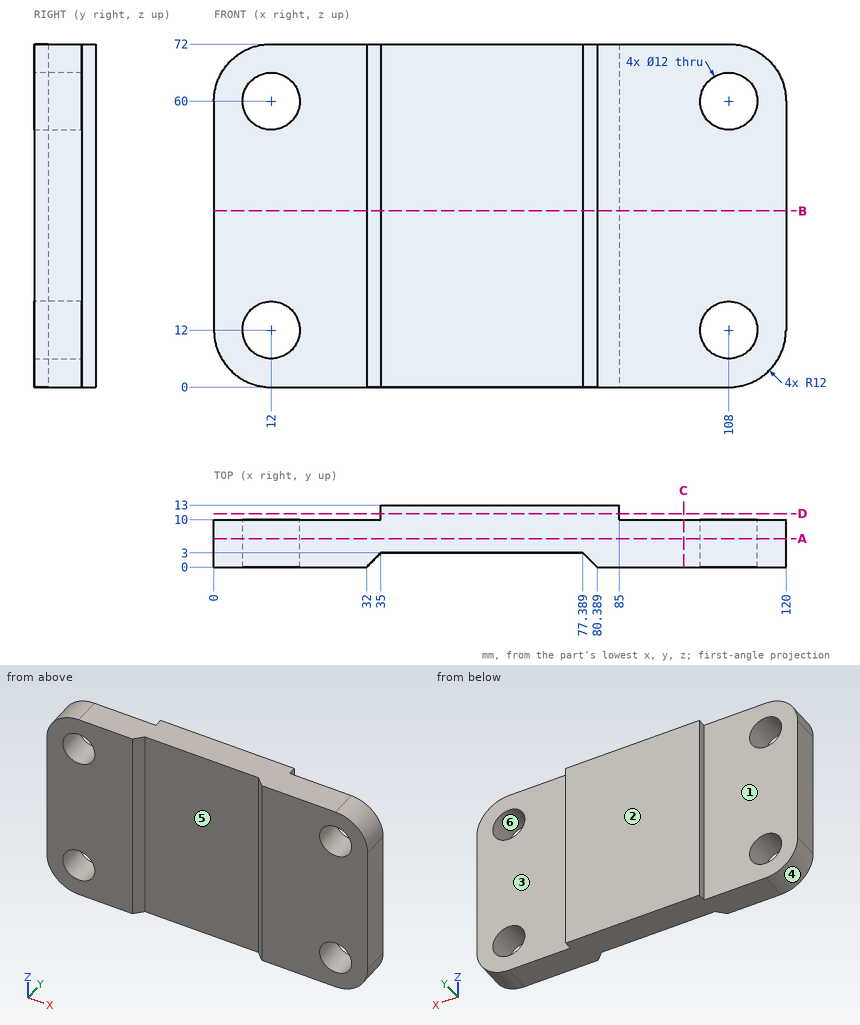
Study the drawing (mm; zero at the part's minimum x, y, z) and answer. A direction names the side the tool comes from. Give positions to 0.01 mm unless a question says otherwise; leave off trailing zeros. Order: outer loops, then holes, each group sorted by start corner. A loop starts at its lowest first (then second) coordinate and runs counter-clockwise, first axis right, second up. Notation, with made-up numbers: (86, -14.75) -> (133, -14.75) arc R23 ccw to (133, 17.25) -> close; hole circle Ø2 at (41, -32.75). An arc over 180 degrees is marked (long way). Write item = value, one per line.
1. A cutting plane is placed at C-C, the plane x = 98.5. Write down the section's boundary in (y, z), and give its area (3 significant figures).
Numbers:
outline = (0, 0) -> (10, 0) -> (10, 72) -> (0, 72) -> close
area = 720 mm²
2. The mould has two halves that part along Z. Classify the marked faces 4, 5 and 6: +Z half, -Z half, draft (parallel to the pull), parting line (faces both ways), or undercut.
Numbers:
face_4 = -Z half
face_5 = draft
face_6 = undercut
3. A cutting plane is placed at D-D, the plane y = 11.25. Write down the section's boundary in (x, z).
Numbers:
outline = (35, 0) -> (85, 0) -> (85, 72) -> (35, 72) -> close
4. A cutting plane is placed at B-B, the plane z = 37. Write down the section's boundary in (x, y), and give its area (3 significant figures).
Numbers:
outline = (0, 0) -> (32, 0) -> (35, 3) -> (77.39, 3) -> (80.39, 0) -> (120, 0) -> (120, 10) -> (85, 10) -> (85, 13) -> (35, 13) -> (35, 10) -> (0, 10) -> close
area = 1,210 mm²
5. Straight lines are drawn through the part: line 1 along Z through (x, y) = (108.5, 3.5); line 2 along Z through (x, y) = (11, 6.5); line 3 along Y through (x, z) = (38, 37.5). For each, find the intervals that lie inside material, in ascending order.
Numbers:
line_1 = 0.01 to 6.02, 17.98 to 54.02, 65.98 to 71.99
line_2 = 0.04 to 6.08, 17.92 to 54.08, 65.92 to 71.96
line_3 = 3 to 13
6. Given pin 1 (9.5 mm diameter, centred on x = 108, z = 60, fed in from -Y); pin 2 (10 mm diameter, centred on x = 63.5, z = 19.5, fed in from -Y); pin 3 (10.5 mm diameter, centred on x = 103, z = 32.5, fed in from +Y), each flat-ended and moving along its own axis, determine where each tip first touches the part or whether it passes through.
Numbers:
pin_1 = through
pin_2 = 3
pin_3 = 10
7. For the marked faces 1, 2 and 3, determine the directions among +Z, -Z, +X, -X, +Y, -Y from which every point of the face is accessible in a straight line to the end or side of a thin tool.
Numbers:
face_1 = +Z, -Z, -X, +Y
face_2 = +Z, -Z, +X, -X, +Y
face_3 = +Z, -Z, +X, +Y
8. A cutting plane is placed at A-A, the plane y = 6. Write down the section's boundary in (x, z).
Numbers:
outline = (0, 12) arc R12 ccw to (12, 0) -> (108, 0) arc R12 ccw to (120, 12) -> (120, 60) arc R12 ccw to (108, 72) -> (12, 72) arc R12 ccw to (0, 60) -> close; hole circle Ø12 at (12, 12); hole circle Ø12 at (12, 60); hole circle Ø12 at (108, 12); hole circle Ø12 at (108, 60)
